Check sheet for the modelled part. Datum: model origin and axes. Units: mm. Coordinates: 2 decimals unless noted, no trailing zeros. Write each loop counter-clockwise with the first axis right and the second up, starting at its lowest first coordinate (ties: lowest second). Pieces come first, ordered by that corner, then holes. Notation, with made-up numbers: (6, 1) - (18, 1) arc R17 cw to (18, 20) - close; hole circle Ø9 at (86.25, 42). An arc over 180 degrees is marked (long way). Use one line per item in the form item = value. Start each with the question number.
1. Draft check along X on faces 1 (the face through (-6.311, 0.626, -26.844)), 2 (the face through (0, 1, -19)), 3 (the face through (-5, 1.27, -19)). Enter one of: +X half, -X half, draft (parallel to the pull), parting line (faces both ways), or undercut.
2. Cross-section at A-A on x = -5.08. Record the boundary of the cut face in (y, z), then the cut area to 3 significant figures.
3. Cross-section at B-B on z = -29.21. Record the boundary of the cut face in (x, y), then the cut area to 3 significant figures.
4. Scan lines: line 1 along Z through (x, y) = (-5.08, 0.35); line 2 along Z through (x, y) = (-4, 0.8); line 3 along X through (y, z) = (0.1, -29). Record each from-to range of solid material in increasing order.
5. Cross-section at C-C on y = 0.4. Record the boundary of the cut face in (x, z).
Autodesk Inventor part; units mm, degrees
ref_plane "YZ Plane" through (0, 0, 0) normal (1, 0, 0) x (0, 1, 0)
ref_plane "XZ Plane" through (0, 0, 0) normal (0, 1, 0) x (-1, 0, 0)
ref_plane "XY Plane" through (0, 0, 0) normal (0, 0, 1) x (1, 0, 0)
sketch "Sketch1" plane through (0, 0, 0) normal (0, 1, 0) x (-1, 0, 0)
  line L0 (0, 0) -> (10.16, 0)
  line L1 (10.16, 0) -> (10.16, -38.1)
  line L2 (10.16, -38.1) -> (0, -38.1)
  line L3 (0, -38.1) -> (0, 0)
  circle A0 centre (5.08, -8.89) radius 2.667
  circle A1 centre (5.08, -29.21) radius 2.667
  point P0 (5.08, -38.1)
  dimension "d0" = 10.16
  dimension "d1" = 38.1
  dimension "d2" = 5.334
  dimension "d3" = 5.334
  dimension "d4" = 5.08
  dimension "d5" = 5.08
  dimension "d6" = 20.32
  dimension "d7" = 8.89
extrude "Extrusion1" add sketch "Sketch1" along normal blind 1.27
properties part number "DrillSpacer"
Final values:
q1.face_1 = undercut
q1.face_2 = +X half
q1.face_3 = draft
q2.outline = (0, -38.1) - (1.27, -38.1) - (1.27, -31.88) - (0, -31.88) - close; (0, -26.54) - (1.27, -26.54) - (1.27, -11.56) - (0, -11.56) - close; (0, -6.22) - (1.27, -6.22) - (1.27, 0) - (0, 0) - close
q2.area = 34.8 mm²
q3.outline = (-10.16, 0) - (-7.75, 0) - (-7.75, 1.27) - (-10.16, 1.27) - close; (-2.41, 0) - (0, 0) - (0, 1.27) - (-2.41, 1.27) - close
q3.area = 6.13 mm²
q4.line_1 = -38.1 to -31.88, -26.54 to -11.56, -6.22 to 0
q4.line_2 = -38.1 to -31.65, -26.77 to -11.33, -6.45 to 0
q4.line_3 = -10.16 to -7.74, -2.42 to 0
q5.outline = (-10.16, -38.1) - (0, -38.1) - (0, 0) - (-10.16, 0) - close; hole circle Ø5.33 at (-5.08, -29.21); hole circle Ø5.33 at (-5.08, -8.89)
